from build123d import *

# Parameters (mm, degrees)
SKETCH1_R           = 2.0193
SKETCH1_R_2         = 14.2875
SKETCH1_R_3         = 9.525
BOSS_EXTRUDE1_DEPTH = 6.35


with BuildPart() as part:
    # Sketch1 → Boss-Extrude1 (new body)
    with BuildSketch(Plane.XY):
        with BuildLine():
            Line((-33.53048127, 8.925931463), (-19.355373509, 35.661972159))
            ThreePointArc((-19.355373509, 35.661972159), (0, 47.3075), (19.355373509, 35.661972159))
            Line((19.355373509, 35.661972159), (33.53048127, 8.925931463))
            ThreePointArc((33.53048127, 8.925931463), (34.598037392, 3.378882244), (32.374264723, -1.813830556))
            ThreePointArc((32.374264723, -1.813830556), (30.688328298, -5.411180272), (31.04222425, -9.368207471))
            ThreePointArc((31.04222425, -9.368207471), (26.679838242, -21.125411227), (14.391737161, -18.62244825))
            ThreePointArc((14.391737161, -18.62244825), (10.500045405, -15.985191191), (5.801286392, -16.133694592))
            ThreePointArc((5.801286392, -16.133694592), (0, -17.145), (-5.801286392, -16.133694592))
            ThreePointArc((-5.801286392, -16.133694592), (-10.500045405, -15.985191191), (-14.391737161, -18.62244825))
            ThreePointArc((-14.391737161, -18.62244825), (-26.679838242, -21.125411227), (-31.04222425, -9.368207471))
            ThreePointArc((-31.04222425, -9.368207471), (-30.688328298, -5.411180272), (-32.374264723, -1.813830556))
            ThreePointArc((-32.374264723, -1.813830556), (-34.598037392, 3.378882244), (-33.53048127, 8.925931463))
        make_face()
        with Locations((25.014116927, 4.410663713)):
            Circle(SKETCH1_R, mode=Mode.SUBTRACT)
        with Locations((21.997045256, -12.7)):
            Circle(SKETCH1_R, mode=Mode.SUBTRACT)
        with Locations((-21.997045256, -12.7)):
            Circle(SKETCH1_R, mode=Mode.SUBTRACT)
        with Locations((-25.014116927, 4.410663713)):
            Circle(SKETCH1_R, mode=Mode.SUBTRACT)
        with Locations((0, 25.4)):
            Circle(SKETCH1_R_2, mode=Mode.SUBTRACT)
        Circle(SKETCH1_R_3, mode=Mode.SUBTRACT)
    extrude(amount=BOSS_EXTRUDE1_DEPTH)


solid = part.part
For this review, take the finished solid that the model builds, in its own axes (mm). Round coordinates to 2 decimals unless told otherwise and drop trailing zeros. Order: outer loops, then holes, each group sorted by start corner. A loop starts at its lowest first (then second) coordinate and runs counter-clockwise, first axis right, second up. Notation, with made-up numbers: M -13.75,77.5 L 11.25,77.5 A7 cw 11.25,82.5 Z; hole C -36.75,-34.5 d8. An arc over 180 degrees is marked long. Use a Markdown table: item, result. Add a question column.
Item 1: Add section A-A, the plane y = -12.7. Give the boundary of the cut face in (x, z), then the cut area to 3 significant figures.
Item 2: Insertion check: pin 1 (3.5 mm diameter, centred on x = -22, y = -12.7, fed in from -Z); pin 2 (3 mm diameter, centred on y = 38, z = 2, fed in from +X); pin 3 (2 mm diameter, centred on x = 25, z = 3.5, fed in from +Y). Each pin has a flat end and moves straight along its axis. Give the tip position at first contact, or say it passes through.
Item 3: To check wall thickness, follow line 1 along X through (y, z) = (-11, 3.75); line 2 along Y through (x, z) = (-1.5, 4.5); line 3 along Y through (x, z) = (5, 0.5). State the ranges of each line that lie inside material, in increasing order.
Item 4: Add section B-B, the plane x = 0. State how many separate pieces and enclosed holes the cut face has, then the cut area to 3 significant figures.
Item 5: Mouldability with a two-part tool opening along X and no side actions: class faces 1 (the cylindrical face through (-34.59, 3.3, 3.13)), 2 (the flat face through (8.2, 5.2, 0)), 3 (the cylindrical face through (26.1, 6.113, 3.131)), 4 (the flat face through (26.344, 22.481, 3.131)) as released by +X, released by -X, zero draft, split by the parting line, or undercut.
Item 6: Add section D-D, the plane y = 0. Give the boundary of the cut face in (x, z) (3 decimals), then the cut area to 3 significant figures.
Geometry results:
| question | item | result |
|---|---|---|
| 1 | outline | M -31.64,0 L -24.02,0 L -24.02,6.35 L -31.64,6.35 Z; M -19.98,0 L 19.98,0 L 19.98,6.35 L -19.98,6.35 Z; M 24.02,0 L 31.64,0 L 31.64,6.35 L 24.02,6.35 Z |
| 1 | area | 350 mm² |
| 2 | pin 1 | passes through |
| 2 | pin 2 | stops at x = 18.89 |
| 2 | pin 3 | stops at y = 26.9 |
| 3 | line 1 | x = -31.49 to -23.09, -20.91 to 20.91, 23.09 to 31.49 |
| 3 | line 2 | y = -17.08 to -9.41, 9.41 to 11.19, 39.61 to 47.26 |
| 3 | line 3 | y = -16.4 to -8.11, 8.11 to 12.02, 38.78 to 46.73 |
| 4 | separate pieces | 3 |
| 4 | enclosed holes | 0 |
| 4 | area | 107 mm² |
| 5 | face 1 | released by -X |
| 5 | face 2 | zero draft |
| 5 | face 3 | undercut |
| 5 | face 4 | released by +X |
| 6 | outline | M -33.585,0 L -9.525,0 L -9.525,6.35 L -33.585,6.35 Z; M 9.525,0 L 33.585,0 L 33.585,6.35 L 9.525,6.35 Z |
| 6 | area | 306 mm² |
